from build123d import *

# Parameters (mm, degrees)
SKETCH1_W                    = 50
SKETCH1_H                    = 7
REVOLVE5_ANGLE               = 167.5
SHELL2_T                     = 3
CUT_EXTRUDE3_DEPTH           = 77.072333999
CUT_EXTRUDE3_DEPTH_BACK      = 10
CUT_EXTRUDE4_DEPTH           = 77.072333999
CUT_EXTRUDE4_DEPTH_BACK      = 10
CUT_EXTRUDE_THIN1_DEPTH      = 77.072333999
CUT_EXTRUDE_THIN1_DEPTH_BACK = 20
CUT_EXTRUDE_THIN2_DEPTH      = 77.072333999
CUT_EXTRUDE_THIN2_DEPTH_BACK = 20
CUT_EXTRUDE_THIN3_DEPTH      = 76.000787866
CUT_EXTRUDE_THIN3_DEPTH_BACK = 20
SKETCH18_R                   = 8
BOSS_EXTRUDE3_DEPTH          = 3


with BuildPart() as part:
    # Sketch1 → Revolve5 (revolve)
    with BuildSketch(Plane(origin=(0, 0, 0), x_dir=(1, 0, 0), z_dir=(0, 1, 0))):
        with Locations((25, 3.5)):
            Rectangle(SKETCH1_W, SKETCH1_H)
    revolve(axis=Axis((0, 0, 0), (0, 0, 1)), revolution_arc=REVOLVE5_ANGLE)

    # Shell2
    shell2_openings = [part.faces().sort_by_distance(p)[0] for p in [
        (25, 0, -3.5),
        (-24.407400178, 5.410990348, -3.5),
    ]]
    offset(amount=SHELL2_T, openings=shell2_openings, kind=Kind.INTERSECTION)

    # Sketch11 → Cut-Extrude3 (cut, two sides: drawn at the far end of the back side and taken through both)
    with BuildSketch(Plane.XY.offset(3).offset(-CUT_EXTRUDE3_DEPTH_BACK)):
        Polygon((-295.067343662, 38.119573796), (-51.743688377, 11.471299539), (53, 0), (296.323655284, -26.648274258), (243.027106769, -513.295584826), (-348.363892177, -448.527736772), align=None)
    extrude(amount=CUT_EXTRUDE3_DEPTH + CUT_EXTRUDE3_DEPTH_BACK, mode=Mode.SUBTRACT)

    # Sketch12 → Cut-Extrude4 (cut, two sides: drawn at the far end of the back side and taken through both)
    with BuildSketch(Plane(origin=(0, 0, -10), x_dir=(-1, 0, 0), z_dir=(0, 0, -1)).offset(-CUT_EXTRUDE4_DEPTH_BACK)):
        Polygon((-296.323655284, -26.648274258), (-53, 0), (51.743688377, 11.471299539), (295.067343662, 38.119573796), (348.363892177, -448.527736772), (-243.027106769, -513.295584826), align=None)
    extrude(amount=CUT_EXTRUDE4_DEPTH + CUT_EXTRUDE4_DEPTH_BACK, mode=Mode.SUBTRACT)

    # Sketch13 → Cut-Extrude-Thin1 (cut, two sides: drawn at the far end of the back side and taken through both)
    with BuildSketch(Plane(origin=(0, 0, -10), x_dir=(-1, 0, 0), z_dir=(0, 0, -1)).offset(-CUT_EXTRUDE_THIN1_DEPTH_BACK)):
        Polygon((48.779244367, 11.146640118), (47.419699991, 23.560551191), (57.360263374, 24.64921994), (58.719807749, 12.235308866), align=None)
    extrude(amount=CUT_EXTRUDE_THIN1_DEPTH + CUT_EXTRUDE_THIN1_DEPTH_BACK, mode=Mode.SUBTRACT)

    # Sketch14 → Cut-Extrude-Thin2 (cut, two sides: drawn at the far end of the back side and taken through both)
    with BuildSketch(Plane(origin=(0, 0, -10), x_dir=(-1, 0, 0), z_dir=(0, 0, -1)).offset(-CUT_EXTRUDE_THIN2_DEPTH_BACK)):
        Polygon((-50.035555989, 0.324659421), (-51.39409796, 12.729417605), (-81.215788107, 9.46341136), (-79.857246136, -2.941346825), align=None)
    extrude(amount=CUT_EXTRUDE_THIN2_DEPTH + CUT_EXTRUDE_THIN2_DEPTH_BACK, mode=Mode.SUBTRACT)

    # Sketch15 → Cut-Extrude-Thin3 (cut, two sides: drawn at the far end of the back side and taken through both)
    with BuildSketch(Plane(origin=(0, 0, -10), x_dir=(-1, 0, 0), z_dir=(0, 0, -1)).offset(-CUT_EXTRUDE_THIN3_DEPTH_BACK)):
        with BuildLine():
            ThreePointArc((-41.982664634, 1.20659446), (-4.572408744, 41.750366205), (40.726353012, 10.264705079))
            Line((40.726353012, 10.264705079), (11.636100861, 2.93277288))
            ThreePointArc((11.636100861, 2.93277288), (-1.306402498, 11.928676059), (-11.995047038, 0.344741274))
            Line((-11.995047038, 0.344741274), (-41.982664634, 1.20659446))
        make_face()
    extrude(amount=CUT_EXTRUDE_THIN3_DEPTH + CUT_EXTRUDE_THIN3_DEPTH_BACK, mode=Mode.SUBTRACT)


with BuildPart() as body_2:
    # of the pieces the cut leaves, the one that is kept (cut_extrude_thin3_keep)
    add(part.part.solids().sort_by_distance((49.998919737, 0.328671743, 0))[0])

    # Sketch18 → Boss-Extrude3 (add)
    with BuildSketch(Plane.XY.offset(3)):
        with Locations((-39.855418013, 18.217155785)):
            Circle(SKETCH18_R)
        with Locations((42.853599633, 9.159045166)):
            Circle(SKETCH18_R)
    extrude(amount=-BOSS_EXTRUDE3_DEPTH)


solid = body_2.part
Geometry: final body of the model. Coordinates: model frame, mm. A direction names the side the tool comes from. Coordinates: 2 decimals unless noted, no trailing zeros. Order: outer loops, then holes, each group sorted by start corner. A loop starts at its lowest first (then second) coordinate and runs counter-clockwise, first axis right, second up.
1) Section C-C (x = 28.5). Return loops of the section in (y, z) (3 decimals).
Result sheet:
outline: (30.85, -10) - (44.685, -10) - (44.685, 3) - (30.85, 3) - (30.85, 0) - (41.082, 0) - (41.082, -7) - (30.85, -7) - close
2) Ray query, probe 1 along Z at (x, y) = (47, 10); probe 2 along X at (y, z) = (22, -1.5); probe 3 along X at (y, z) = (12, -3). Return the intervals inside material, ascending.
Result sheet:
probe 1: z = -10 to -7, 0 to 3
probe 2: x = -47.59 to -44.9, 44.9 to 48.22
probe 3: x = -48.69 to -48.54, 48.54 to 51.31
3) Section A-A (y = 47.5). Return loops of the section in (x, z), then the cut area to 3 significant figures.
Result sheet:
outline: (-23.51, -10) - (23.51, -10) - (23.51, 3) - (-23.51, 3) - close; hole (-15.61, -7) - (15.61, -7) - (15.61, 0) - (-15.61, 0) - close
area: 393 mm2
4) First-contact query: P1, Ø2, axis at x = 33, z = 1.5, coming from the +Y side; P2, Ø3, axis at y = 22.5, z = -5.5, coming from the +X side; P3, Ø6, axis at x = 33.5, z = -4.5, coming from the +Y side. Flat tips, straight axial feed; report the tip coordinate or a pass-through.
Result sheet:
P1: stops at y = 42.25
P2: stops at x = 48.66
P3: stops at y = 43.34
5) Draft query along Z for faces 1 (the cylindrical face through (-32.64, 14.76, 1.52)), 2 (the flat face through (1.1, 42.4, 3)), 3 (the flat face through (5, 44, -7)). Return one class per face: released by +Z, released by -Z, zero draft, split by the parting line, or undercut.
Result sheet:
face 1: zero draft
face 2: released by +Z
face 3: undercut
6) Section B-B (y = 31). Return loops of the section in (x, z).
Result sheet:
outline: (-42.99, -10) - (-28.34, -10) - (-28.34, -7) - (-39.23, -7) - (-39.23, 0) - (-28.34, 0) - (-28.34, 3) - (-42.99, 3) - close; (28.34, -10) - (42.99, -10) - (42.99, 3) - (28.34, 3) - (28.34, 0) - (39.23, 0) - (39.23, -7) - (28.34, -7) - close
7) Set-up query: faces 4 (the cylindrical face through (5.41, 41.65, -8.48)), 5 (the cylindrical face through (6.455, 49.582, -3.549)), 6 (the cylindrical face through (35.002, 7.624, 1.521)). Return all of +Z, -Z, +X, -X, +Y, -Y with unobstructed straight access to the full face (end or side cutting, diameter ignored); none if empty.
Result sheet:
face 4: -Z, -Y
face 5: -Y
face 6: +Z, -Z
